```python
from build123d import *

# Parameters (mm, degrees)
SKETCH1_R           = 24
SKETCH1_R_2         = 19
BOSS_EXTRUDE1_DEPTH = 2.5
SKETCH2_R           = 24
BOSS_EXTRUDE2_DEPTH = 2
SKETCH3_R           = 2.5
CUT_EXTRUDE1_DEPTH  = 35.238136632


with BuildPart() as part:
    # Sketch1 → Boss-Extrude1 (new body)
    with BuildSketch(Plane(origin=(0, 0, 0), x_dir=(1, 0, 0), z_dir=(0, 1, 0))):
        with Locations(Location((0, 0, 0), (0, 0, 270))):
            Circle(SKETCH1_R)
        with Locations(Location((0, 0, 0), (0, 0, 270))):
            Circle(SKETCH1_R_2, mode=Mode.SUBTRACT)
    extrude(amount=BOSS_EXTRUDE1_DEPTH)

    # Sketch2 → Boss-Extrude2 (add)
    with BuildSketch(Plane(origin=(0, 2.5, 0), x_dir=(1, 0, 0), z_dir=(0, 1, 0))):
        with Locations(Location((0, 0, 0), (0, 0, 270))):
            Circle(SKETCH2_R)
    extrude(amount=BOSS_EXTRUDE2_DEPTH)

    # Sketch3 → Cut-Extrude1 (cut, through all)
    with BuildSketch(Plane.XZ):
        with Locations(Location((0, 0, 0), (0, 0, 270))):
            Circle(SKETCH3_R)
    extrude(amount=-CUT_EXTRUDE1_DEPTH, mode=Mode.SUBTRACT)


solid = part.part
```
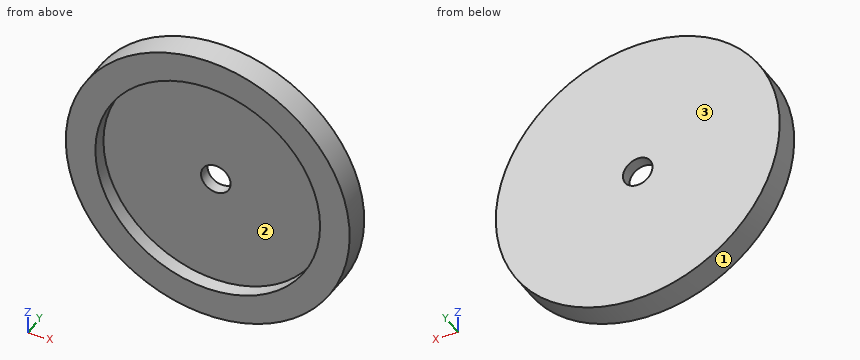
CAD build for the part. Positions are in the model's coordinates, mm. Face numbers are marked on the shaded views. Round coordinates to 2 decimals unless told otherwise and drop trailing zeros. Order: outer loops, then holes, each group sorted by start corner. A loop starts at its lowest first (then second) coordinate and runs counter-clockwise, first axis right, second up. Notation, with made-up numbers: (-23.5, -7) - (11.5, -7) arc R5 ccw to (11.5, 0) - close; hole circle Ø11 at (44.25, 59.25). An arc over 180 degrees is marked (long way). Answer in a Markdown table with one row per item. Add a question column.
(1) Probe L1, parallel to X at y = 3.8, z = 0; L2, parallel to X at y = 1.4, z = 0; L3, parallel to Y at x = 1.5, z = 9. List the from-to ranges inside material, lowest first. Write a range as [from, to].
(2) Mould opens along X. For the marked faces 1, 2 and 3 say: +X half, -X half, draft (parallel to the pull), parting line (faces both ways), or undercut.
(3) Band-saw the part on D-D on z = 8. List the corners of the cut face in (x, y).
(4) Band-saw the part on C-C on x = -6. List the corners of the cut face in (y, z).
(5) Band-saw the part on A-A on x = 0. List the corners of the cut face in (y, z).
(6) Band-saw the part on B-B on z = 0. List the corners of the cut face in (x, y).
(7) Drop flat-ended pins along their axis: pin 1 Ø2 at (y, z) = (0.5, -15) entering from +X; pin 2 Ø1 at (y, z) = (3.5, -17.5) entering from +X; pin 3 Ø8 at (x, z) = (4.5, 7.5) entering from -Y. Give the stop position or say it passes through.
Data:
| question | item | result |
|---|---|---|
| 1 | L1 | x = [-24, -2.5], [2.5, 24] |
| 1 | L2 | x = [-24, -19], [19, 24] |
| 1 | L3 | y = [2.5, 4.5] |
| 2 | face 1 | parting line |
| 2 | face 2 | undercut |
| 2 | face 3 | draft |
| 3 | outline | (-22.63, 0) - (-17.23, 0) - (-17.23, 2.5) - (17.23, 2.5) - (17.23, 0) - (22.63, 0) - (22.63, 4.5) - (-22.63, 4.5) - close |
| 4 | outline | (0, -23.24) - (4.5, -23.24) - (4.5, 23.24) - (0, 23.24) - (0, 18.03) - (2.5, 18.03) - (2.5, -18.03) - (0, -18.03) - close |
| 5 | outline | (0, -24) - (4.5, -24) - (4.5, -2.5) - (2.5, -2.5) - (2.5, -19) - (0, -19) - close; (0, 19) - (2.5, 19) - (2.5, 2.5) - (4.5, 2.5) - (4.5, 24) - (0, 24) - close |
| 6 | outline | (-24, 0) - (-19, 0) - (-19, 2.5) - (-2.5, 2.5) - (-2.5, 4.5) - (-24, 4.5) - close; (2.5, 2.5) - (19, 2.5) - (19, 0) - (24, 0) - (24, 4.5) - (2.5, 4.5) - close |
| 7 | pin 1 | stops at x = 19.49 |
| 7 | pin 2 | stops at x = 16.94 |
| 7 | pin 3 | stops at y = 2.5 |
